Geometry check sheet. Reference: the model listing, model coordinates, mm. A direction names the side the tool comes from. Give positions to 0.01 mm unless a question says otherwise; leave off trailing zeros. Order: outer loops, then holes, each group sorted by start corner. A loop starts at its lowest first (then second) coordinate and runs counter-clockwise, first axis right, second up. Notation, with made-up numbers: M -18.5,64 L 23.5,64 A37 cw 23.5,103 Z; hole C 14,32.25 d5. An arc over 180 degrees is marked long. Answer as CSV lines item,"result". Start each with the question number.
Q1. Set-up check for faces 1 (the flat face through (-86, -34.007, 2)), 2 (the flat face through (-68, -7, 0)): record each of +Z, -Z, +X, -X, +Y, -Y from which the full face is reachable in a straight line by a thin tool's end or side.
Q2. Mould release check, pull along Y, two halves, no side actions. Record for faces 3 (the flat face through (-68, -7, 5)), 4 (the flat face through (-83.267, 7, 2)), 5 (the flat face through (-78, -8.636, 2)): +Y half, -Y half, draft (parallel to the pull), parting line (faces both ways), or undercut.
Q3. Section check D-D, the plane x = -26.5. Record the boundary of the cut face in (y, z).
Q4. Go/stop test with a flat-tipped pin: pin 1 (1.9 mm diameter, centred on x = -116.12, y = -38.2, fed in from -Z). Record where the tip stops, or that it passes through.
Q5. Section check B-B, the plane y = 7.5. Record the boundary of the cut face in (x, z), then the cut area to 3 significant figures.
Q6. Thickness scan on line 1 (Y direction, x = -84, z = 4); line 2 (X direction, y = 4.5, z = 3.6); line 3 (X direction, y = -23.5, z = 2.55). Record the ranges inside material, lowest first.
Q7. Section check C-C, the plane x = -46. Record the boundary of the cut face in (y, z).
Q8. Section check A-A, the plane y = -18. Record the boundary of the cut face in (x, z).
Autodesk Inventor part; units mm, degrees
ref_plane "YZ Plane" through (0, 0, 0) normal (1, 0, 0) x (0, 1, 0)
ref_plane "XZ Plane" through (0, 0, 0) normal (0, 1, 0) x (-1, 0, 0)
ref_plane "XY Plane" through (0, 0, 0) normal (0, 0, 1) x (1, 0, 0)
sketch "Boceto1" plane through (0, 0, 0) normal (0, 0, 1) x (1, 0, 0)
  arc A0 (-116.1173, 21.3488) -> (-117.6673, 19.7988) centre (-116.1173, 19.7988) ccw
  arc A1 (-117.6673, 19.7988) -> (-116.1173, 18.2488) centre (-116.1173, 19.7988) ccw
  arc A2 (-116.1173, 18.2488) -> (-114.5673, 19.7988) centre (-116.1173, 19.7988) ccw
  arc A3 (-114.5673, 19.7988) -> (-116.1173, 21.3488) centre (-116.1173, 19.7988) ccw
  arc A4 (-67.1173, 21.3488) -> (-68.6673, 19.7988) centre (-67.1173, 19.7988) ccw
  arc A5 (-68.6673, 19.7988) -> (-67.1173, 18.2488) centre (-67.1173, 19.7988) ccw
  arc A6 (-67.1173, 18.2488) -> (-65.5673, 19.7988) centre (-67.1173, 19.7988) ccw
  arc A7 (-65.5673, 19.7988) -> (-67.1173, 21.3488) centre (-67.1173, 19.7988) ccw
  arc A8 (-18.1173, 21.3488) -> (-19.6673, 19.7988) centre (-18.1173, 19.7988) ccw
  arc A9 (-19.6673, 19.7988) -> (-18.1173, 18.2488) centre (-18.1173, 19.7988) ccw
  arc A10 (-18.1173, 18.2488) -> (-16.5673, 19.7988) centre (-18.1173, 19.7988) ccw
  arc A11 (-16.5673, 19.7988) -> (-18.1173, 21.3488) centre (-18.1173, 19.7988) ccw
  arc A12 (-18.1173, -7.6512) -> (-19.6673, -9.2012) centre (-18.1173, -9.2012) ccw
  arc A13 (-19.6673, -9.2012) -> (-18.1173, -10.7512) centre (-18.1173, -9.2012) ccw
  arc A14 (-18.1173, -10.7512) -> (-16.5673, -9.2012) centre (-18.1173, -9.2012) ccw
  arc A15 (-16.5673, -9.2012) -> (-18.1173, -7.6512) centre (-18.1173, -9.2012) ccw
  arc A16 (-67.1173, -7.6512) -> (-68.6673, -9.2012) centre (-67.1173, -9.2012) ccw
  arc A17 (-68.6673, -9.2012) -> (-67.1173, -10.7512) centre (-67.1173, -9.2012) ccw
  arc A18 (-67.1173, -10.7512) -> (-65.5673, -9.2012) centre (-67.1173, -9.2012) ccw
  arc A19 (-65.5673, -9.2012) -> (-67.1173, -7.6512) centre (-67.1173, -9.2012) ccw
  arc A20 (-116.1173, -7.6512) -> (-117.6673, -9.2012) centre (-116.1173, -9.2012) ccw
  arc A21 (-117.6673, -9.2012) -> (-116.1173, -10.7512) centre (-116.1173, -9.2012) ccw
  arc A22 (-116.1173, -10.7512) -> (-114.5673, -9.2012) centre (-116.1173, -9.2012) ccw
  arc A23 (-114.5673, -9.2012) -> (-116.1173, -7.6512) centre (-116.1173, -9.2012) ccw
  arc A24 (-116.1173, -36.6512) -> (-117.6673, -38.2012) centre (-116.1173, -38.2012) ccw
  arc A25 (-117.6673, -38.2012) -> (-116.1173, -39.7512) centre (-116.1173, -38.2012) ccw
  arc A26 (-116.1173, -39.7512) -> (-114.5673, -38.2012) centre (-116.1173, -38.2012) ccw
  arc A27 (-114.5673, -38.2012) -> (-116.1173, -36.6512) centre (-116.1173, -38.2012) ccw
  arc A28 (-18.1173, -36.6512) -> (-19.6673, -38.2012) centre (-18.1173, -38.2012) ccw
  arc A29 (-19.6673, -38.2012) -> (-18.1173, -39.7512) centre (-18.1173, -38.2012) ccw
  arc A30 (-18.1173, -39.7512) -> (-16.5673, -38.2012) centre (-18.1173, -38.2012) ccw
  arc A31 (-16.5673, -38.2012) -> (-18.1173, -36.6512) centre (-18.1173, -38.2012) ccw
  arc A32 (-107.1173, -22.7762) -> (-112.0423, -27.7012) centre (-107.1173, -27.7012) ccw
  arc A33 (-112.0423, -27.7012) -> (-107.1173, -32.6262) centre (-107.1173, -27.7012) ccw
  arc A34 (-107.1173, -32.6262) -> (-102.1923, -27.7012) centre (-107.1173, -27.7012) ccw
  arc A35 (-102.1923, -27.7012) -> (-107.1173, -22.7762) centre (-107.1173, -27.7012) ccw
  arc A36 (-27.1173, -22.7762) -> (-32.0423, -27.7012) centre (-27.1173, -27.7012) ccw
  arc A37 (-32.0423, -27.7012) -> (-27.1173, -32.6262) centre (-27.1173, -27.7012) ccw
  arc A38 (-27.1173, -32.6262) -> (-22.1923, -27.7012) centre (-27.1173, -27.7012) ccw
  arc A39 (-22.1923, -27.7012) -> (-27.1173, -22.7762) centre (-27.1173, -27.7012) ccw
  arc A40 (-77.8673, -23.1512) -> (-79.4173, -24.7012) centre (-77.8673, -24.7012) ccw
  arc A41 (-79.4173, -24.7012) -> (-77.8673, -26.2512) centre (-77.8673, -24.7012) ccw
  arc A42 (-77.8673, -26.2512) -> (-76.3173, -24.7012) centre (-77.8673, -24.7012) ccw
  arc A43 (-76.3173, -24.7012) -> (-77.8673, -23.1512) centre (-77.8673, -24.7012) ccw
  line L0 (-111.9673, 1.9488) -> (-83.2673, 1.9488)
  line L1 (-83.2673, 1.9488) -> (-83.2673, 12.6488)
  line L2 (-83.2673, 12.6488) -> (-111.9673, 12.6488)
  line L3 (-111.9673, 12.6488) -> (-111.9673, 1.9488)
  line L4 (-50.9673, 12.6488) -> (-50.9673, 1.9488)
  line L5 (-50.9673, 1.9488) -> (-22.2673, 1.9488)
  line L6 (-22.2673, 1.9488) -> (-22.2673, 12.6488)
  line L7 (-22.2673, 12.6488) -> (-50.9673, 12.6488)
  line L8 (-80.7673, -16.563) -> (-81.6794, -15.5552)
  line L9 (-81.6794, -15.5552) -> (-91.0552, -15.5552)
  line L10 (-91.0552, -15.5552) -> (-91.9673, -16.563)
  line L11 (-91.9673, -16.563) -> (-91.9673, -34.0068)
  line L12 (-91.9673, -34.0068) -> (-80.7673, -34.0068)
  line L13 (-80.7673, -34.0068) -> (-80.7673, -16.563)
  line L14 (-11.9023, 27.5138) -> (-122.3323, 27.5138)
  line L15 (-122.3323, 27.5138) -> (-122.3323, -42.9162)
  line L16 (-122.3323, -42.9162) -> (-11.9023, -42.9162)
  line L17 (-11.9023, -42.9162) -> (-11.9023, 27.5138)
  line L18 (-75.3023, -14.7662) -> (-75.3023, -8.6362)
  line L19 (-75.3023, -8.6362) -> (-80.4323, -8.6362)
  line L20 (-80.4323, -8.6362) -> (-80.4323, -14.7662)
  line L21 (-80.4323, -14.7662) -> (-75.3023, -14.7662)
  line L22 (-80.4323, -34.6362) -> (-80.4323, -40.7662)
  line L23 (-80.4323, -40.7662) -> (-75.3023, -40.7662)
  line L24 (-75.3023, -40.7662) -> (-75.3023, -34.6362)
  line L25 (-75.3023, -34.6362) -> (-80.4323, -34.6362)
  point P0 (0, 0)
extrude "Extrusión1" add sketch "Boceto1" along normal blind 5
properties part number "carro x lado motor pieza 4"
Answer block:
1,face 1,"+Z, -Z"
1,face 2,"-Z, +X, -X, +Y, -Y"
2,face 3,"draft"
2,face 4,"undercut"
2,face 5,"undercut"
3,outline,"M -42.92,0 L -32.59,0 L -32.59,5 L -42.92,5 Z; M -22.82,0 L 1.95,0 L 1.95,5 L -22.82,5 Z; M 12.65,0 L 27.51,0 L 27.51,5 L 12.65,5 Z"
4,pin 1,"passes through"
5,outline,"M -122.33,0 L -111.97,0 L -111.97,5 L -122.33,5 Z; M -83.27,0 L -50.97,0 L -50.97,5 L -83.27,5 Z; M -22.27,0 L -11.9,0 L -11.9,5 L -22.27,5 Z"
5,area,"265 mm2"
6,line 1,"y = -42.92 to -34.01, -15.56 to 1.95, 12.65 to 27.51"
6,line 2,"x = -122.33 to -111.97, -83.27 to -50.97, -22.27 to -11.9"
6,line 3,"x = -122.33 to -109.69, -104.55 to -91.97, -80.77 to -78.85, -76.89 to -29.69, -24.55 to -11.9"
7,outline,"M -42.92,0 L 1.95,0 L 1.95,5 L -42.92,5 Z; M 12.65,0 L 27.51,0 L 27.51,5 L 12.65,5 Z"
8,outline,"M -122.33,0 L -91.97,0 L -91.97,5 L -122.33,5 Z; M -80.77,0 L -11.9,0 L -11.9,5 L -80.77,5 Z"
